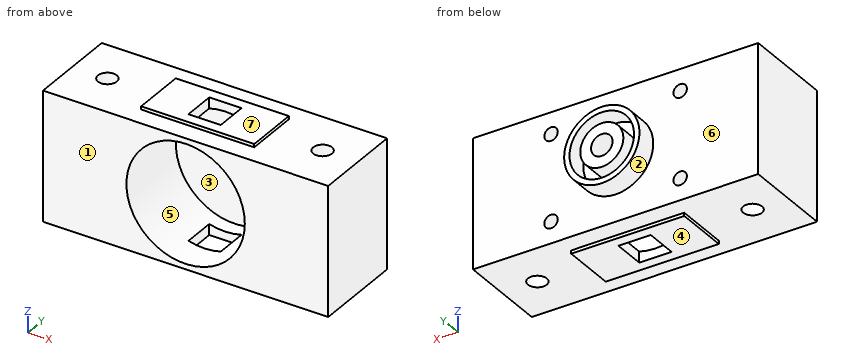
```python
from build123d import *

# Parameters (mm, degrees)
SKETCH_1_R          = 1.75
EXTRUDE_1_DEPTH     = 12
SKETCH_3_R          = 2
CUT_EXTRUDE_1_DEPTH = 18
SKETCH_4_W          = 22.4
SKETCH_4_H          = 14.3
SKETCH_4_W_2        = 6
SKETCH_4_H_2        = 6
EXTRUDE_2_DEPTH     = 1.2
SKETCH_5_W          = 21
SKETCH_5_H          = 10
SKETCH_5_W_2        = 6
SKETCH_5_H_2        = 6
EXTRUDE_3_DEPTH     = 0.6
SKETCH_14_W         = 24.4
SKETCH_14_H         = 23.6
EXTRUDE_6_DEPTH     = 14.3
CUT_EXTRUDE_START   = 2.7
SKETCH_12_R         = 11
CUT_EXTRUDE_6_DEPTH = 14.3
SKETCH_15_W         = 6
SKETCH_15_H         = 6
CUT_EXTRUDE_7_DEPTH = 25.4
SKETCH_6_R          = 7
SKETCH_6_R_2        = 6
SKETCH_6_R_3        = 4
SKETCH_6_R_4        = 2
EXTRUDE_4_DEPTH     = 4
M3X0_51_D           = 2.5
M3X0_51_DEPTH       = 11.5
M3X0_51_TIP         = 0.751075774


with BuildPart() as part:
    # Sketch 1 → Extrude 1 (new body, symmetric)
    with BuildSketch(Plane.XY):
        Polygon((11.2, -17), (11.2, -2.7), (0, -2.7), (0, 0), (26.5, 0), (26.5, -17), align=None)
        with Locations((20, -8.5)):
            Circle(SKETCH_1_R, mode=Mode.SUBTRACT)
    extrude_1 = extrude(amount=EXTRUDE_1_DEPTH, both=True)

    # Mirror 1: Extrude 1 across plane
    add(extrude_1.mirror(Plane(origin=(0, -2.7, -12), x_dir=(0, 0, 1), z_dir=(-1, 0, 0))))

    # Sketch 3 → Cut-Extrude 1 (cut, through all)
    with BuildSketch(Plane(origin=(0, 0, 0), x_dir=(1, 0, 0), z_dir=(0, 1, 0))):
        Circle(SKETCH_3_R)
    extrude(amount=-CUT_EXTRUDE_1_DEPTH, mode=Mode.SUBTRACT)

    # Sketch 4 → Extrude 2 (add)
    with BuildSketch(Plane(origin=(0, 0, -12), x_dir=(-1, 0, 0), z_dir=(0, 0, -1))):
        with Locations((0, -9.85)):
            Rectangle(SKETCH_4_W, SKETCH_4_H)
        with Locations((0, -8.5)):
            Rectangle(SKETCH_4_W_2, SKETCH_4_H_2, mode=Mode.SUBTRACT)
    extrude_2 = extrude(amount=-EXTRUDE_2_DEPTH)

    # Sketch 5 → Extrude 3 (add)
    with BuildSketch(Plane(origin=(0, 0, -12), x_dir=(-1, 0, 0), z_dir=(0, 0, -1))):
        with Locations((0, -8.5)):
            Rectangle(SKETCH_5_W, SKETCH_5_H)
        with Locations((0, -8.5)):
            Rectangle(SKETCH_5_W_2, SKETCH_5_H_2, mode=Mode.SUBTRACT)
    extrude_3 = extrude(amount=EXTRUDE_3_DEPTH)

    # Mirror 2: Extrude 2, Extrude 3 across plane
    add(extrude_2.mirror(Plane.XY))
    add(extrude_3.mirror(Plane.XY))

    # Sketch 14 → Extrude 6 (add)
    with BuildSketch(Plane.XZ.offset(2.7)):
        Rectangle(SKETCH_14_W, SKETCH_14_H)
    extrude(amount=EXTRUDE_6_DEPTH)

    # Sketch 12 → Cut-Extrude 6 (cut)
    with BuildSketch(Plane.XZ.offset(CUT_EXTRUDE_START)):
        Circle(SKETCH_12_R)
    extrude(amount=CUT_EXTRUDE_6_DEPTH, mode=Mode.SUBTRACT)

    # Sketch 15 → Cut-Extrude 7 (cut, through all)
    with BuildSketch(Plane.XY.offset(11.8)):
        with Locations((0, -8.5)):
            Rectangle(SKETCH_15_W, SKETCH_15_H)
    extrude(amount=-CUT_EXTRUDE_7_DEPTH, mode=Mode.SUBTRACT)

    # Sketch 6 → Extrude 4 (add)
    with BuildSketch(Plane(origin=(0, 0, 0), x_dir=(1, 0, 0), z_dir=(0, 1, 0))):
        Circle(SKETCH_6_R)
        Circle(SKETCH_6_R_2, mode=Mode.SUBTRACT)
        Circle(SKETCH_6_R_3)
        Circle(SKETCH_6_R_4, mode=Mode.SUBTRACT)
    extrude(amount=EXTRUDE_4_DEPTH)

    # M3x0.51
    with Locations(Plane(origin=(0, 0, 0), x_dir=(1, 0, 0), z_dir=(0, 1, 0))):
        with Locations((12, 8), (12, -8), (-12, -8), (-12, 8)):
            Hole(M3X0_51_D / 2, depth=M3X0_51_DEPTH)
            with Locations((0, 0, -(M3X0_51_DEPTH + M3X0_51_TIP / 2))):  # 118° drill point
                Cone(0, M3X0_51_D / 2, M3X0_51_TIP, mode=Mode.SUBTRACT)


solid = part.part
```
Read the model definition and answer for the solid it produces. Units are mm, in the model's axes. Face numbers are marked on the shaded views. A direction names the side the tool comes from. Round coordinates to 2 decimals unless told otherwise and drop trailing zeros. Write each loop counter-clockwise with the first axis right and the second up, starting at its lowest first coordinate (ties: lowest second). Pieces come first, ordered by that corner, then holes. Notation, with made-up numbers: M 42,35 L 97,35 A17 cw 97,68 Z; hole C -32,25.25 d9. An arc over 180 degrees is marked long. One line per item, written item: value.
Q1. Find section D-D on z = -2.5. Write down the section's boundary in (x, y), plus the area to 3 significant figures.
Data:
outline: M -26.5,-17 L -10.71,-17 L -10.71,-2.7 L 10.71,-2.7 L 10.71,-17 L 26.5,-17 L 26.5,0 L 6.54,0 L 6.54,4 L 5.45,4 L 5.45,0 L 3.12,0 L 3.12,4 L -3.12,4 L -3.12,0 L -5.45,0 L -5.45,4 L -6.54,4 L -6.54,0 L -26.5,0 Z; hole C -20,-8.5 d3.5; hole C 20,-8.5 d3.5
area: 609 mm2
Q2. Which of the six approach directions +Z, -Z, +X, -X, +Y, -Y give full straight-line access (tool end or side, diameter ignored) to the marked faces 5, 6 and 7?
Data:
face 5: -Y
face 6: +Y
face 7: +Z, +X, -X, +Y, -Y
Q3. For a pull along Z with two mould halves and no side action, classify the marked faces 1, 2, 3 and 4 as +Z half, -Z half, draft (parallel to the pull), parting line (faces both ways), or undercut.
Data:
face 1: draft
face 2: parting line
face 3: undercut
face 4: -Z half
Q4. Flat-ended cylindrical pins translate along their axes: pin 1 Ø1 at (x, z) = (1, 12) entering from +Y; pin 2 Ø2 at (x, y) = (-18, -2.5) entering from -Z; pin 3 Ø3 at (x, y) = (-1, -14) entering from +Z; pin 4 Ø2 at (x, z) = (-12, -8) entering from +Y. Find the tip coordinate at first contact, or state that the pin passes through.
Data:
pin 1: y = 0
pin 2: z = -12
pin 3: z = 12.6
pin 4: y = -11.65
Q5. Straight lines are drawn through the part: line 1 (Z direction, x = -12, y = -3.75); line 2 (Z direction, x = 0, y = 1.3); line 3 (Y direction, x = 20, z = 4.5). For each, find the intervals that lie inside material, in ascending order. Write a range as [from, to].
Data:
line 1: [-12, -9.25], [-6.75, 6.75], [9.25, 12]
line 2: [-7, -6], [-4, -2], [2, 4], [6, 7]
line 3: [-17, -10.25], [-6.75, 0]
Q6. Find section A-A on y = -8.5. Count the separate pieces of the cut face and the enclosed holes in it, plus the area to 3 significant figures.
Data:
separate pieces: 4
enclosed holes: 4
area: 709 mm2
Q7. Find section B-B on x = 20. Write down the section's boundary in (y, z).
Data:
outline: M -17,-12 L -10.25,-12 L -10.25,12 L -17,12 Z; M -6.75,-12 L 0,-12 L 0,12 L -6.75,12 Z
Q8. Find section C-C on z = 1. Write down the section's boundary in (x, y).
Data:
outline: M -26.5,-17 L -10.95,-17 L -10.95,-2.7 L -1.73,-2.7 L -1.73,4 L -3.87,4 L -3.87,0 L -5.92,0 L -5.92,4 L -6.93,4 L -6.93,0 L -26.5,0 Z; M 1.73,-2.7 L 10.95,-2.7 L 10.95,-17 L 26.5,-17 L 26.5,0 L 6.93,0 L 6.93,4 L 5.92,4 L 5.92,0 L 3.87,0 L 3.87,4 L 1.73,4 Z; hole C -20,-8.5 d3.5; hole C 20,-8.5 d3.5
